Source: CAD feature listing. Evaluate the final solid. Frame: model axes, mm. Face numbers are marked on the shaded views. A direction names the side the tool comes from. Give positions to 0.01 mm unless a question says otherwise; leave off trailing zeros. Write each loop counter-clockwise with the first axis right and the second up, starting at its lowest first coordinate (ties: lowest second). Pieces come first, ordered by that corner, then holes. Notation, with made-up numbers: (-9.5, -22.5) -> (43.5, -22.5) arc R28 ccw to (43.5, 4.5) -> close; hole circle Ø6 at (13.25, -37). An arc over 180 degrees is marked (long way). Answer as a JSON object with one key per item and string values. Group by question number.
Item 1: Pull-direction query (X, two-part tool) for the marked faces 1, 2 and 3; classes: pulls with the +X half, pulls with the -X half, needs draft (parallel to the pull), parting line crosses it, or undercut.
Item 2: First-contact query: pin 1 Ø6.5 at (x, y) = (1, -20) entering from +Z; pin 2 Ø2.5 at (x, z) = (-29.5, 22.5) entering from -Y; pin 3 Ø6 at (x, z) = (7, 19) entering from -Y; pin 4 Ø0.8 at (y, z) = (4.5, 18) entering from -X. Flat tips, straight axial feed; report the tip coordinate or a pass-through.
Item 3: Section query D-D on y = -9. Return the cut outline in (x, z).
Item 4: Section query C-C on z = 20.75. Return the cut outline in (x, y).
Item 5: Section query B-B on x = 0. Return the cut outline in (y, z).
Item 6: Ray query, probe 1 along X at (y, z) = (-3.5, 24.5); probe 2 along X at (y, z) = (3, 20.5); probe 3 along Z at (x, y) = (16, 4). Return the intervals inside material, ascending. Write a range as from..to.
Item 7: Section query A-A on y = 21.3. Return the cut outline in (x, z).
Item 8: Access query for the marked faces 4 and 5. Directions: +Z, -Z, +X, -X, +Y, -Y. A direction counts if a zero-diameter tool reaches every point of the face in a straight line with its end or side. Return the directions, or none.
from build123d import *

# Parameters (mm, degrees)
F2_DEPTH = 1.6
F1_R     = 3
F1_W     = 3
F1_H     = 13.5
F1_H_2   = 11.6
F1_R_2   = 1.1303
F1_H_3   = 1.5
F3_DEPTH = 9
F4_DEPTH = 3
F5_DEPTH = 5
F6_DEPTH = 6.35
F7_R     = 3
F8_DEPTH = 3.5


with BuildPart() as f2:
    # F1 (on offset) → F2 (new body)
    with BuildSketch(Plane.XY.offset(18.75)):
        Polygon((28.1, -9.8), (30.6, -9.8), (30.6, 9.8), (28.1, 9.8), (28.1, 0), align=None)
    extrude(amount=-F2_DEPTH)

    # F1 (on offset) → F3 (join)
    with BuildSketch(Plane.XY.offset(18.75)):
        Polygon((-14.6, -13.3), (22.6, -13.3), (22.6, -10.3), (22.6, 10.3), (22.6, 13.3), (-14.6, 13.3), align=None)
        Polygon((-27.6, -13.3), (-14.6, -13.3), (-14.6, 13.3), (-27.6, 13.3), (-27.6, 1.7), (-27.6, -11.8), align=None)
        with BuildLine():
            Line((3.1063091707, -25.2848662841), (30.6, -16.3))
            Line((30.6, -16.3), (-30.6, -16.3))
            Line((-30.6, -16.3), (-3.1063091707, -25.2848662841))
            ThreePointArc((-3.1063091707, -25.2848662841), (0, -25.7795602219), (3.1063091707, -25.2848662841))
        make_face()
        with Locations((0, -21.3)):
            Circle(F1_R, mode=Mode.SUBTRACT)
        with BuildLine():
            Line((-30.6, 16.3), (30.6, 16.3))
            Line((30.6, 16.3), (3.1063091707, 25.2848662841))
            ThreePointArc((3.1063091707, 25.2848662841), (0, 25.7795602219), (-3.1063091707, 25.2848662841))
            Line((-3.1063091707, 25.2848662841), (-30.6, 16.3))
        make_face()
        with Locations((0, 21.3)):
            Circle(F1_R, mode=Mode.SUBTRACT)
        Polygon((27.6, -10.3), (27.6, -13.3), (22.6, -13.3), (-14.6, -13.3), (-27.6, -13.3), (-30.6, -13.3), (-30.6, -16.3), (30.6, -16.3), (30.6, -10.3), align=None)
        Polygon((27.6, 13.3), (27.6, 10.3), (30.6, 10.3), (30.6, 16.3), (-30.6, 16.3), (-30.6, 13.3), (-27.6, 13.3), (-14.6, 13.3), (22.6, 13.3), align=None)
        Polygon((22.6, -13.3), (27.6, -13.3), (27.6, -10.3), (27.6, 10.3), (27.6, 13.3), (22.6, 13.3), (22.6, 10.3), (22.6, -10.3), align=None)
        Polygon((28.1, -9.8), (30.6, -9.8), (30.6, 9.8), (28.1, 9.8), (28.1, 0), align=None)
        with Locations((-29.1, -5.05)):
            Rectangle(F1_W, F1_H)
        with Locations((-29.1, 7.5)):
            Rectangle(F1_W, F1_H_2)
        with Locations((0, 21.3)):
            Circle(F1_R)
        with Locations((0, 21.3)):
            Circle(F1_R_2, mode=Mode.SUBTRACT)
        with Locations((0, -21.3)):
            Circle(F1_R)
        with Locations((0, -21.3)):
            Circle(F1_R_2, mode=Mode.SUBTRACT)
        Polygon((27.6, 10.3), (27.6, -10.3), (30.6, -10.3), (30.6, -9.8), (28.1, -9.8), (28.1, 0), (28.1, 9.8), (30.6, 9.8), (30.6, 10.3), align=None)
        with Locations((-29.1, -12.55)):
            Rectangle(F1_W, F1_H_3)
        with Locations((0, -21.3)):
            Circle(F1_R_2)
    extrude(amount=F3_DEPTH)

    # F1 (on offset) → F4 (cut)
    with BuildSketch(Plane.XY.offset(18.75)):
        Polygon((-14.6, -13.3), (22.6, -13.3), (22.6, -10.3), (22.6, 10.3), (22.6, 13.3), (-14.6, 13.3), align=None)
        with Locations((0, -21.3)):
            Circle(F1_R_2)
    extrude(amount=F4_DEPTH, mode=Mode.SUBTRACT)

    # F1 (on offset) → F5 (cut)
    with BuildSketch(Plane.XY.offset(18.75)):
        with Locations((-29.1, -5.05)):
            Rectangle(F1_W, F1_H)
        with Locations((0, -21.3)):
            Circle(F1_R_2)
    extrude(amount=F5_DEPTH, mode=Mode.SUBTRACT)

    # F1 (on offset) → F6 (cut)
    with BuildSketch(Plane.XY.offset(18.75)):
        Polygon((-27.6, -13.3), (-14.6, -13.3), (-14.6, 13.3), (-27.6, 13.3), (-27.6, 1.7), (-27.6, -11.8), align=None)
        with Locations((0, -21.3)):
            Circle(F1_R_2)
    extrude(amount=F6_DEPTH, mode=Mode.SUBTRACT)

    # F7 (on face) → F8 (cut)
    with BuildSketch(Plane.XY.offset(27.75)):
        with Locations((0, 21.3)):
            Circle(F7_R)
        with Locations((0, -21.3)):
            Circle(F7_R)
    extrude(amount=-F8_DEPTH, mode=Mode.SUBTRACT)


solid = f2.part
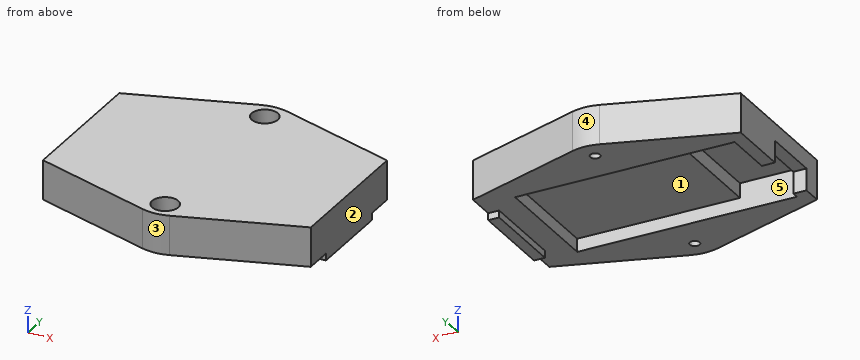
Worked answers:
{
 "1": {"face 1": "undercut", "face 2": "pulls with the +X half", "face 3": "parting line crosses it"},
 "2": {"pin 1": "z = 27.75", "pin 2": "y = -17.07", "pin 3": "y = -24.99", "pin 4": "x = 28.1"},
 "3": {"outline": "(-30.6, 23.75) -> (-27.6, 23.75) -> (-27.6, 25.1) -> (-14.6, 25.1) -> (-14.6, 21.75) -> (22.6, 21.75) -> (22.6, 18.75) -> (28.1, 18.75) -> (28.1, 17.15) -> (30.6, 17.15) -> (30.6, 27.75) -> (-30.6, 27.75) -> close"},
 "4": {"outline": "(-30.6, -16.3) -> (-3.11, -25.28) arc R10 ccw to (3.11, -25.28) -> (30.6, -16.3) -> (30.6, 16.3) -> (3.11, 25.28) arc R10 ccw to (-3.11, 25.28) -> (-30.6, 16.3) -> (-30.6, 1.7) -> (-27.6, 1.7) -> (-27.6, 13.3) -> (22.6, 13.3) -> (22.6, -13.3) -> (-27.6, -13.3) -> (-27.6, -11.8) -> (-30.6, -11.8) -> close; hole circle Ø2.26 at (0, -21.3); hole circle Ø2.26 at (0, 21.3)"},
 "5": {"outline": "(-25.78, 18.75) -> (-22.43, 18.75) -> (-22.43, 24.25) -> (-24.3, 24.25) -> (-24.3, 27.75) -> (-25.78, 27.75) -> close; (-20.17, 18.75) -> (-13.3, 18.75) -> (-13.3, 21.75) -> (13.3, 21.75) -> (13.3, 18.75) -> (20.17, 18.75) -> (20.17, 24.25) -> (18.3, 24.25) -> (18.3, 27.75) -> (-18.3, 27.75) -> (-18.3, 24.25) -> (-20.17, 24.25) -> close; (22.43, 18.75) -> (25.78, 18.75) -> (25.78, 27.75) -> (24.3, 27.75) -> (24.3, 24.25) -> (22.43, 24.25) -> close"},
 "6": {"probe 1": "-30.6..-27.6, -14.6..30.6", "probe 2": "-30.6..-27.6, 22.6..30.6", "probe 3": "21.75..27.75"},
 "7": {"outline": "(-15.3, 18.75) -> (-1.13, 18.75) -> (-1.13, 24.25) -> (-3, 24.25) -> (-3, 27.75) -> (-15.3, 27.75) -> close; (1.13, 18.75) -> (15.3, 18.75) -> (15.3, 27.75) -> (3, 27.75) -> (3, 24.25) -> (1.13, 24.25) -> close"},
 "8": {"face 4": "+Z, -Z, +Y", "face 5": "-Z"}
}
